```python
from build123d import *

# Parameters (mm, degrees)
SKETCH1_W           = 440
SKETCH1_H           = 175
SKETCH1_R           = 9.5
SKETCH1_R_2         = 1.75
SKETCH1_R_3         = 1.65
SKETCH1_R_4         = 1.15
SKETCH1_R_5         = 3.25
SKETCH1_R_6         = 2.25
SKETCH1_W_2         = 27.7
SKETCH1_H_2         = 20
SKETCH1_W_3         = 10
SKETCH1_H_3         = 8.5
BOSS_EXTRUDE1_DEPTH = 3


with BuildPart() as part:
    # Sketch1 → Boss-Extrude1 (new body)
    with BuildSketch(Plane.XY):
        with Locations((220, 87.5)):
            Rectangle(SKETCH1_W, SKETCH1_H)
        with Locations((125, 50)):
            Circle(SKETCH1_R, mode=Mode.SUBTRACT)
        with Locations((115.5, 62)):
            Circle(SKETCH1_R_2, mode=Mode.SUBTRACT)
        with Locations((134.5, 38)):
            Circle(SKETCH1_R_2, mode=Mode.SUBTRACT)
        with Locations((285, 50)):
            Circle(SKETCH1_R_3, mode=Mode.SUBTRACT)
        with Locations((325, 50)):
            Circle(SKETCH1_R_3, mode=Mode.SUBTRACT)
        with Locations((387.5, 60)):
            Circle(SKETCH1_R_4, mode=Mode.SUBTRACT)
        with Locations((376, 50)):
            Circle(SKETCH1_R_2, mode=Mode.SUBTRACT)
        with Locations((399, 50)):
            Circle(SKETCH1_R_2, mode=Mode.SUBTRACT)
        with Locations((10, 165)):
            Circle(SKETCH1_R_5, mode=Mode.SUBTRACT)
        with Locations((10, 10)):
            Circle(SKETCH1_R_5, mode=Mode.SUBTRACT)
        with Locations((430, 10)):
            Circle(SKETCH1_R_5, mode=Mode.SUBTRACT)
        with Locations((430, 165)):
            Circle(SKETCH1_R_5, mode=Mode.SUBTRACT)
        with Locations((202.5, 134.5)):
            Circle(SKETCH1_R_6, mode=Mode.SUBTRACT)
        with Locations((202.5, 97.5)):
            Circle(SKETCH1_R_6, mode=Mode.SUBTRACT)
        with Locations((237.5, 134.5)):
            Circle(SKETCH1_R_6, mode=Mode.SUBTRACT)
        with Locations((237.5, 97.5)):
            Circle(SKETCH1_R_6, mode=Mode.SUBTRACT)
        with Locations((237.5, 77.5)):
            Circle(SKETCH1_R_6, mode=Mode.SUBTRACT)
        with Locations((237.5, 40.5)):
            Circle(SKETCH1_R_6, mode=Mode.SUBTRACT)
        with Locations((202.5, 77.5)):
            Circle(SKETCH1_R_6, mode=Mode.SUBTRACT)
        with Locations((202.5, 40.5)):
            Circle(SKETCH1_R_6, mode=Mode.SUBTRACT)
        with Locations((305, 50)):
            Rectangle(SKETCH1_W_2, SKETCH1_H_2, mode=Mode.SUBTRACT)
        with Locations((387.5, 50)):
            Rectangle(SKETCH1_W_3, SKETCH1_H_3, mode=Mode.SUBTRACT)
    extrude(amount=BOSS_EXTRUDE1_DEPTH)


solid = part.part
```
CAD build for the part. Positions are in the model's coordinates, mm. Coordinates: 2 decimals unless noted, no trailing zeros. Order: outer loops, then holes, each group sorted by start corner. A loop starts at its lowest first (then second) coordinate and runs counter-clockwise, first axis right, second up. Notation, with made-up numbers: (-11, 33) - (46, 33) arc R23 ccw to (46, 53) - close; hole circle Ø6 at (58.5, 17). An arc over 180 degrees is marked (long way). Answer in a Markdown table with one row per item.
1. Drill centre lines: L1, parallel to Y at x = 387.5, z = 0.9; L2, parallel to Y at x = 202.5, z = 2.35; L3, parallel to X at y = 41.5, z = 0.45. Where is each one in solid material? Low to high. Write a range as from..to.
Answer:
| item | result |
|---|---|
| L1 | 0..45.75, 54.25..58.85, 61.15..175 |
| L2 | 0..38.25, 42.75..75.25, 79.75..95.25, 99.75..132.25, 136.75..175 |
| L3 | 0..120.76, 129.24..200.48, 204.52..235.48, 239.52..291.15, 318.85..440 |
2. Slice it at A-A, the plane x = 297. List the corners of the cut face in (y, z), then the cut area to 3 significant figures.
Answer:
| item | result |
|---|---|
| outline | (0, 0) - (40, 0) - (40, 3) - (0, 3) - close; (60, 0) - (175, 0) - (175, 3) - (60, 3) - close |
| area | 465 mm² |
3. Pull direction Y, two halves, no side cores. Call faces 1 (the face through (130.11, 58.01, 1.48)), 2 (the face through (217, 89, 0)): +Y half, -Y half, draft (parallel to the pull), parting line (faces both ways), or undercut.
Answer:
| item | result |
|---|---|
| face 1 | undercut |
| face 2 | draft |
4. Slice it at B-B, the plane z = 1.6. Give the number of separate pieces and of enclosed holes in the cut face, then the cut area to 3 significant figures.
Answer:
| item | result |
|---|---|
| separate pieces | 1 |
| enclosed holes | 22 |
| area | 75,800 mm² |
